Geometry check sheet. Reference: the model listing, model coordinates, mm. Face numbers are marked on the shaded views. A direction names the side the tool comes from. Coordinates: 2 decimals unless noted, no trailing zeros. Order: outer loops, then holes, each group sorted by start corner. A loop starts at its lowest first (then second) coordinate and runs counter-clockwise, first axis right, second up. Notation, with made-up numbers: (-34, 22) -> (7, 22) arc R5 ccw to (7, 26) -> close; hole circle Ø11 at (-25.5, 25.25). An arc over 180 degrees is marked (long way). Answer in a Markdown table with one row per item. Add a question column.
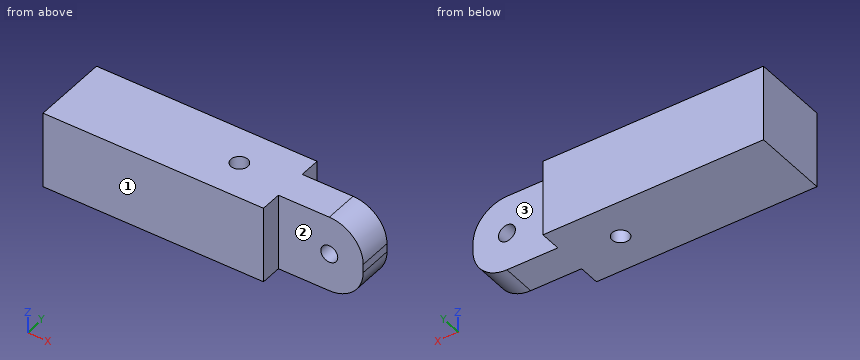
```python
from build123d import *

# Parameters (mm, degrees)
F0_W     = 45
F0_H     = 45
F1_DEPTH = 65
F2_R     = 5
F3_DEPTH = 45.001
F4_W     = 20
F4_H     = 45
F5_DEPTH = 50
F6_R     = 20
F7_R     = 5
F8_DEPTH = 25


with BuildPart() as f1:
    # F0 (on Right) → F1 (new body, symmetric)
    with BuildSketch(Plane.YZ):
        with Locations((-22.5, 22.5)):
            Rectangle(F0_W, F0_H)
    extrude(amount=F1_DEPTH, both=True)

    # F2 (on face) → F3 (cut, through all)
    with BuildSketch(Plane.XY.offset(45)):
        with Locations((35, -22.5)):
            Circle(F2_R)
    extrude(amount=-F3_DEPTH, mode=Mode.SUBTRACT)

    # F4 (on face) → F5 (join)
    with BuildSketch(Plane.YZ.offset(65)):
        with Locations((-22.5, 22.5)):
            Rectangle(F4_W, F4_H)
    extrude(amount=F5_DEPTH)

    # F6
    f6_edges = [f1.edges().sort_by_distance(p)[0] for p in [
        (115, -22.5, 45),
        (115, -22.5, 0),
    ]]
    fillet(f6_edges, radius=F6_R)

    # F7 (on face) → F8 (cut)
    with BuildSketch(Plane.XZ.offset(32.5)):
        with Locations((95, 22.5)):
            Circle(F7_R)
    extrude(amount=-F8_DEPTH, mode=Mode.SUBTRACT)


solid = f1.part
```
(1) Scan lines: line 1 along Y through (x, z) = (35, 16); line 2 along Z through (x, y) = (95, -17.75); line 3 along X through (y, z) = (-20, 22). Record each from-to range of solid material in increasing order.
(2) Go/stop test with flat-tipped pins: P1, Ø4, axis at y = -9, z = 14.5, coming from the +X side; P2, Ø1.5, axis at y = -14, z = 39, coming from the +X side. Record where each tip stops, or that it passes through.
(3) Cross-section at A-A (z = 22.5). Enter the section's corners in (x, y), plus the area to 3 significant figures.
(4) Cross-section at D-D (z = 37.5). Enter the section's corners in (x, y).
(5) Access from +Z, -Z, +X, -X, +Y, -Y to the whole of each face (thin tool, end or side, straight path). Record for the marked faces 1, 2 and 3.
(6) Cross-section at C-C (x = 35). Enter the section's corners in (y, z), plus the area to 4 significant figures.
(7) Cross-section at B-B (y = -22.5). Enter the section's corners in (x, z), plus the area to 3 significant figures.
Checks:
| question | item | result |
|---|---|---|
| 1 | line 1 | -45 to -27.5, -17.5 to 0 |
| 1 | line 2 | 0 to 17.5, 27.5 to 45 |
| 1 | line 3 | -65 to 30.67, 39.33 to 90.03, 99.97 to 115 |
| 2 | P1 | x = 65 |
| 2 | P2 | x = 109.98 |
| 3 | outline | (-65, -45) -> (65, -45) -> (65, -32.5) -> (90, -32.5) -> (90, -12.5) -> (65, -12.5) -> (65, 0) -> (-65, 0) -> close; (100, -32.5) -> (115, -32.5) -> (115, -12.5) -> (100, -12.5) -> close; hole circle Ø10 at (35, -22.5) |
| 3 | area | 6,570 mm² |
| 4 | outline | (-65, -45) -> (65, -45) -> (65, -32.5) -> (110.61, -32.5) -> (110.61, -12.5) -> (65, -12.5) -> (65, 0) -> (-65, 0) -> close; hole circle Ø10 at (35, -22.5) |
| 5 | face 1 | +Z, -Z, +X, -X, -Y |
| 5 | face 2 | +Z, -Z, +X, -Y |
| 5 | face 3 | +Z, -Z, +X, +Y |
| 6 | outline | (-45, 0) -> (-27.5, 0) -> (-27.5, 45) -> (-45, 45) -> close; (-17.5, 0) -> (0, 0) -> (0, 45) -> (-17.5, 45) -> close |
| 6 | area | 1,575 mm² |
| 7 | outline | (-65, 0) -> (30, 0) -> (30, 45) -> (-65, 45) -> close; (40, 0) -> (95, 0) arc R20 ccw to (115, 20) -> (115, 25) arc R20 ccw to (95, 45) -> (40, 45) -> close; hole circle Ø10 at (95, 22.5) |
| 7 | area | 7,400 mm² |
